Part model, mm, in its own coordinate system. Face numbers are marked on the shaded views. A direction names the side the tool comes from. Coordinates: 2 decimals unless noted, no trailing zeros. Write each loop counter-clockwise with the first axis right and the second up, starting at its lowest first coordinate (ties: lowest second). Pieces come first, ordered by that corner, then holes. Notation, with made-up numbers: (51.25, 81.5) -> (86.25, 81.5) arc R30 ccw to (86.25, 104.5) -> close; hole circle Ø8 at (11, 6). An arc over 180 degrees is marked (long way). Write item = value, one per line. Start each with the question number.
Q1. Band-saw the part on A-A, the plane x = -29. List the corners of the cut face in (y, z).
Q2. Probe line 1 (Z direction, x = -29, y = 10); line 2 (Y direction, x = 28.5, z = -7.5). List the from-to ranges inside material, lowest first.
Q3. Band-saw the part on B-B, the plane x = -6.5. List the corners of the cut face in (y, z).
Q4. Tool access for the marked faces 4, 5 and 6: list every direction of +Z, -Z, +X, -X, +Y, -Y with a clear straight run to the whole face (end or side of a thin tool).
Q5. Pull direction X, two halves, no side cores. Call the marked faces 1, 2 and 3: released by +X, released by -X, zero draft, split by the parting line, or undercut.
Q6. Band-saw the part on C-C, the plane z = 31.5. List the corners of the cut face in (x, y).
Q7. Pin check, flat tips, straight feed: P1, Ø4, axis at y = 30.16, z = 27.5, coming from the +X side; P2, Ø5, axis at x = 0, z = 0, coming from the +Y side; P3, Ø3, axis at y = 10.16, z = 27.5, coming from the -X side. Stop position of each tip, or through.
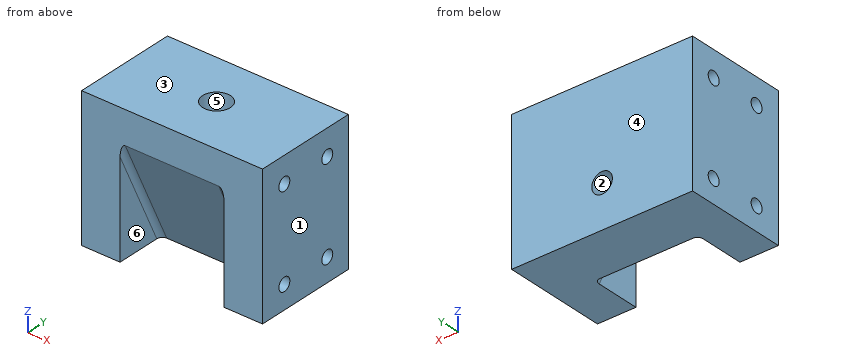
from build123d import *

# Parameters (mm, degrees)
SKETCH1_W                        = 69.6
SKETCH1_H                        = 75
BOSS_EXTRUDE1_DEPTH              = 40
SKETCH3_W                        = 126.991899018
SKETCH3_H                        = 42.64725952
CUT_EXTRUDE2_DEPTH               = 41
F_3_8_16_TAPPED_HOLE1_D          = 7.9375
F_3_8_16_TAPPED_HOLE1_DEPTH      = 15.875
F_3_8_16_TAPPED_HOLE1_TIP        = 2.384665582
F_1_4_20_TAPPED_HOLE1_AT_2_COUNT = 2
F_1_4_20_TAPPED_HOLE1_AT_2_PITCH = 20
F_1_4_20_TAPPED_HOLE1_AT_3_COUNT = 2
F_1_4_20_TAPPED_HOLE1_AT_3_PITCH = 40.311288741
F_1_4_20_TAPPED_HOLE1_AT_4_COUNT = 2
F_1_4_20_TAPPED_HOLE1_AT_4_PITCH = 35
CUT_EXTRUDE3_DEPTH               = 20
F_1_2_13_TAPPED_HOLE1_D          = 10.71626
F_1_2_13_TAPPED_HOLE1_DEPTH      = 25
F_1_2_13_TAPPED_HOLE1_TIP        = 3.219489309
FILLET1_R                        = 2


with BuildPart() as part:
    # Sketch1 → Boss-Extrude1 (new body)
    with BuildSketch(Plane(origin=(0, 0, 0), x_dir=(1, 0, 0), z_dir=(0, 1, 0))):
        Rectangle(SKETCH1_W, SKETCH1_H)
    extrude(amount=BOSS_EXTRUDE1_DEPTH)

    # Sketch3 → Cut-Extrude2 (cut, through all)
    with BuildSketch(Plane(origin=(0, 0, 0), x_dir=(1, 0, 0), z_dir=(0, 1, 0))):
        with Locations((-9.204742755, 37.82362976)):
            Rectangle(SKETCH3_W, SKETCH3_H)
    extrude(amount=CUT_EXTRUDE2_DEPTH, mode=Mode.SUBTRACT)

    # 3/8-16 Tapped Hole1
    with Locations(Plane(origin=(0, 40, 0), x_dir=(1, 0, 0), z_dir=(0, 1, 0))):
        with Locations((0, 0)):
            Hole(F_3_8_16_TAPPED_HOLE1_D / 2, depth=F_3_8_16_TAPPED_HOLE1_DEPTH)
            with Locations((0, 0, -(F_3_8_16_TAPPED_HOLE1_DEPTH + F_3_8_16_TAPPED_HOLE1_TIP / 2))):  # 118° drill point
                Cone(0, F_3_8_16_TAPPED_HOLE1_D / 2, F_3_8_16_TAPPED_HOLE1_TIP, mode=Mode.SUBTRACT)

    # Sketch10 → 1/4-20 Tapped Hole1 (revolve, cut)
    with BuildSketch(Plane(origin=(34.8, 30.16, -7.5), x_dir=(0, 0, -1), z_dir=(0, 1, 0))):
        Polygon((0, 0), (0, 14.533816902), (2.5527, 13), (2.5527, 0), align=None)
    f_1_4_20_tapped_hole1 = revolve(axis=Axis((41.15, 30.16, -7.5), (-1, 0, 0)), mode=Mode.SUBTRACT)

    # 1/4-20 Tapped Hole1 at 2: 1/4-20 Tapped Hole1 ×2
    with Locations(*[(0, -i * F_1_4_20_TAPPED_HOLE1_AT_2_PITCH, 0) for i in range(1, F_1_4_20_TAPPED_HOLE1_AT_2_COUNT)]):
        add(f_1_4_20_tapped_hole1, mode=Mode.SUBTRACT)

    # 1/4-20 Tapped Hole1 at 3: 1/4-20 Tapped Hole1 ×2
    with Locations(*[Vector(0, -0.496138938, 0.868243142) * (i * F_1_4_20_TAPPED_HOLE1_AT_3_PITCH) for i in range(1, F_1_4_20_TAPPED_HOLE1_AT_3_COUNT)]):
        add(f_1_4_20_tapped_hole1, mode=Mode.SUBTRACT)

    # 1/4-20 Tapped Hole1 at 4: 1/4-20 Tapped Hole1 ×2
    with Locations(*[(0, 0, i * F_1_4_20_TAPPED_HOLE1_AT_4_PITCH) for i in range(1, F_1_4_20_TAPPED_HOLE1_AT_4_COUNT)]):
        add(f_1_4_20_tapped_hole1, mode=Mode.SUBTRACT)

    # Mirror1: 1/4-20 Tapped Hole1 across plane
    add(f_1_4_20_tapped_hole1.mirror(Plane(origin=(0, 0, 0), x_dir=(0, 0, 1), z_dir=(1, 0, 0))), mode=Mode.SUBTRACT)

    # Mirror1 copy 1 sketch → Mirror1 copy 1 (revolve, cut)
    with BuildSketch(Plane(origin=(-34.8, 10.16, -7.5), x_dir=(0, 0, -1), z_dir=(0, 1, 0))):
        Polygon((0, 0), (0, -14.533816902), (2.5527, -13), (2.5527, 0), align=None)
    revolve(axis=Axis((-41.15, 10.16, -7.5), (-1, 0, 0)), mode=Mode.SUBTRACT)

    # Mirror1 copy 2 sketch → Mirror1 copy 2 (revolve, cut)
    with BuildSketch(Plane(origin=(-34.8, 10.16, 27.5), x_dir=(0, 0, -1), z_dir=(0, 1, 0))):
        Polygon((0, 0), (0, -14.533816902), (2.5527, -13), (2.5527, 0), align=None)
    revolve(axis=Axis((-41.15, 10.16, 27.5), (-1, 0, 0)), mode=Mode.SUBTRACT)

    # Mirror1 copy 3 sketch → Mirror1 copy 3 (revolve, cut)
    with BuildSketch(Plane(origin=(-34.8, 30.16, 27.5), x_dir=(0, 0, -1), z_dir=(0, 1, 0))):
        Polygon((0, 0), (0, -14.533816902), (2.5527, -13), (2.5527, 0), align=None)
    revolve(axis=Axis((-41.15, 30.16, 27.5), (-1, 0, 0)), mode=Mode.SUBTRACT)

    # Sketch11 → Cut-Extrude3 (cut, symmetric)
    with BuildSketch(Plane(origin=(0, 0, 0), x_dir=(0, 0, -1), z_dir=(1, 0, 0))):
        Polygon((20.112673013, 20.996619633), (-33.5, -4.003380367), (20.112673013, -4.003380367), align=None)
    extrude(amount=CUT_EXTRUDE3_DEPTH, both=True, mode=Mode.SUBTRACT)

    # 1/2-13 Tapped Hole1
    with Locations(Plane.XY.offset(37.5)):
        with Locations((0, 20.718863156)):
            Hole(F_1_2_13_TAPPED_HOLE1_D / 2, depth=F_1_2_13_TAPPED_HOLE1_DEPTH)
            with Locations((0, 0, -(F_1_2_13_TAPPED_HOLE1_DEPTH + F_1_2_13_TAPPED_HOLE1_TIP / 2))):  # 118° drill point
                Cone(0, F_1_2_13_TAPPED_HOLE1_D / 2, F_1_2_13_TAPPED_HOLE1_TIP, mode=Mode.SUBTRACT)

    # Fillet1
    fillet1_edges = [part.edges().sort_by_distance(p)[0] for p in [
        (-20, 9.65600127, 4.207361549),
        (20, 9.65600127, 4.207361549),
    ]]
    fillet(fillet1_edges, radius=FILLET1_R)


solid = part.part
Ans:
q1.outline = (0, -16.5) -> (40, -16.5) -> (40, 37.5) -> (0, 37.5) -> close; hole circle Ø5.11 at (10.16, -7.5); hole circle Ø5.11 at (10.16, 27.5); hole circle Ø5.11 at (30.16, -7.5); hole circle Ø5.11 at (30.16, 27.5)
q2.line_1 = -16.5 to -10.05, -4.95 to 24.95, 30.05 to 37.5
q2.line_2 = 0 to 7.61, 12.71 to 27.61, 32.71 to 40
q3.outline = (0, 24.91) -> (19.31, -16.5) -> (40, -16.5) -> (40, 37.5) -> (0, 37.5) -> close
q4.face_4 = +Z, -Z, +X, -X, +Y
q4.face_5 = +Z
q4.face_6 = -Z, -Y
q5.face_1 = released by +X
q5.face_2 = undercut
q5.face_3 = zero draft
q6.outline = (-34.8, 0) -> (34.8, 0) -> (34.8, 40) -> (-34.8, 40) -> close; hole circle Ø10.72 at (0, 20.72)
q7.P1 = 21.47
q7.P2 = 23.24
q7.P3 = -21.17
